Geometry: final body of the model. Coordinates: model frame, mm. A direction names the side the tool comes from. Coordinates: 2 decimals unless noted, no trailing zeros. Loops run counter-clockwise (first coordinate to the right, second up) from the corner with the lowest first, then second, coordinate; pieces in that order, holes last. Notation, with made-up numbers: M 22,89.5 L 36,89.5 A20 cw 36,125.5 Z; hole C -24,-10 d5. An arc over 180 degrees is marked long. Write item = value, one per line. Start each with the question number.
```python
from build123d import *

# Parameters (mm, degrees)
SKETCH005_AS_DRAWN_R                 = 10
EXTRUDE005_DEPTH                     = 5
EXTRUDE005_ONTO_SKETCH005_ROLL_ANGLE = 90
SKETCH001_AS_DRAWN_W                 = 40
SKETCH001_AS_DRAWN_H                 = 70
SKETCH001_AS_DRAWN_R                 = 3.5
EXTRUDE002_DEPTH                     = 12
EXTRUDE002_ONTO_SKETCH001_ROLL_ANGLE = 90
SKETCH004_AS_DRAWN_R                 = 8.5
SKETCH004_AS_DRAWN_R_2               = 3.5
EXTRUDE004_DEPTH                     = 2
EXTRUDE004_ONTO_SKETCH004_ROLL_ANGLE = 90
SKETCH003_AS_DRAWN_R                 = 5.95
SKETCH003_AS_DRAWN_R_2               = 4
EXTRUDE003_DEPTH                     = 25
EXTRUDE003_ONTO_SKETCH003_ROLL_ANGLE = 90
CYLINDER001_R                        = 16.25
CYLINDER001_DEPTH                    = 10
SKETCH_R                             = 14
EXTRUDE_DEPTH                        = 13
CYLINDER_R                           = 16.25
CYLINDER_DEPTH                       = 10
EXTRUDE001_DEPTH                     = 13


with BuildPart() as contra_nut_cut:
    # Sketch005 as drawn → Extrude005 (new)
    with BuildSketch(Plane.XY):
        Circle(SKETCH005_AS_DRAWN_R)
    extrude(amount=-EXTRUDE005_DEPTH)


with BuildPart() as contra_nut_cut_1:
    # Extrude005 onto Sketch005 roll: moved
    add(contra_nut_cut.part.rotate(Axis((0, 0, 0), (1, 0, 0)), EXTRUDE005_ONTO_SKETCH005_ROLL_ANGLE))


with BuildPart() as contra_nut_cut_2:
    # Extrude005 onto Sketch005 placement: moved
    add(contra_nut_cut_1.part)


with BuildPart() as contra_nut_cut_3:
    # Extrude005 placement: moved
    add(contra_nut_cut_2.part.moved(Location((0, 7, 0))))


with BuildPart() as nut_cut:
    # Sketch001 as drawn → Extrude002 (new)
    with BuildSketch(Plane.XY):
        Rectangle(SKETCH001_AS_DRAWN_W, SKETCH001_AS_DRAWN_H)
        Circle(SKETCH001_AS_DRAWN_R, mode=Mode.SUBTRACT)
    extrude(amount=-EXTRUDE002_DEPTH)


with BuildPart() as nut_cut_1:
    # Extrude002 onto Sketch001 roll: moved
    add(nut_cut.part.rotate(Axis((0, 0, 0), (1, 0, 0)), EXTRUDE002_ONTO_SKETCH001_ROLL_ANGLE))


with BuildPart() as nut_cut_2:
    # Extrude002 onto Sketch001 placement: moved
    add(nut_cut_1.part)

    # Cut002: cut contra-nut-cut
    add(contra_nut_cut_3.part, mode=Mode.SUBTRACT)


with BuildPart() as nut_cut_3:
    # Cut002 placement: moved
    add(nut_cut_2.part.moved(Location((0, -36, 0))))


with BuildPart() as z_bearings_pad:
    # Sketch004 as drawn → Extrude004 (new)
    with BuildSketch(Plane.XY):
        Circle(SKETCH004_AS_DRAWN_R)
        Circle(SKETCH004_AS_DRAWN_R_2, mode=Mode.SUBTRACT)
    extrude(amount=-EXTRUDE004_DEPTH)


with BuildPart() as z_bearings_pad_1:
    # Extrude004 onto Sketch004 roll: moved
    add(z_bearings_pad.part.rotate(Axis((0, 0, 0), (1, 0, 0)), EXTRUDE004_ONTO_SKETCH004_ROLL_ANGLE))


with BuildPart() as z_bearings_pad_2:
    # Extrude004 onto Sketch004 placement: moved
    add(z_bearings_pad_1.part)


with BuildPart() as z_bearings_pad_3:
    # Extrude004 placement: moved
    add(z_bearings_pad_2.part.moved(Location((0, -38, 0))))


with BuildPart() as z_bearings_cylinder:
    # Sketch003 as drawn → Extrude003 (new)
    with BuildSketch(Plane.XY):
        Circle(SKETCH003_AS_DRAWN_R)
        Circle(SKETCH003_AS_DRAWN_R_2, mode=Mode.SUBTRACT)
    extrude(amount=-EXTRUDE003_DEPTH)


with BuildPart() as z_bearings_cylinder_1:
    # Extrude003 onto Sketch003 roll: moved
    add(z_bearings_cylinder.part.rotate(Axis((0, 0, 0), (1, 0, 0)), EXTRUDE003_ONTO_SKETCH003_ROLL_ANGLE))


with BuildPart() as z_bearings_cylinder_2:
    # Extrude003 onto Sketch003 placement: moved
    add(z_bearings_cylinder_1.part)


with BuildPart() as z_bearings_cylinder_3:
    # Extrude003 placement: moved
    add(z_bearings_cylinder_2.part.moved(Location((0, -61, 0))))


with BuildPart() as cylinder001:
    # Cylinder001 → Cylinder001 (new body)
    with BuildSketch(Plane.XY.offset(3)):
        Circle(CYLINDER001_R)
    extrude(amount=CYLINDER001_DEPTH)


with BuildPart() as bearing_nest_r_cut:
    # Sketch → Extrude (new body)
    with BuildSketch(Plane.XY):
        with BuildLine():
            ThreePointArc((20, 0), (0, 20), (-20, 0))
            Line((-20, 0), (-20, -36))
            Line((-20, -36), (20, -36))
            Line((20, -36), (20, 0))
        make_face()
        Circle(SKETCH_R, mode=Mode.SUBTRACT)
    extrude(amount=EXTRUDE_DEPTH)

    # Cut001: cut Cylinder001
    add(cylinder001.part, mode=Mode.SUBTRACT)


with BuildPart() as bearing_nest_r_cut_1:
    # Cut001 placement: moved
    add(bearing_nest_r_cut.part.moved(Location((0, 0, 22))))


with BuildPart() as cylinder:
    # Cylinder → Cylinder (new body)
    with BuildSketch(Plane.XY):
        Circle(CYLINDER_R)
    extrude(amount=CYLINDER_DEPTH)


with BuildPart() as fusion:
    # Sketch → Extrude001 (new body)
    with BuildSketch(Plane.XY):
        with BuildLine():
            ThreePointArc((20, 0), (0, 20), (-20, 0))
            Line((-20, 0), (-20, -36))
            Line((-20, -36), (20, -36))
            Line((20, -36), (20, 0))
        make_face()
        Circle(SKETCH_R, mode=Mode.SUBTRACT)
    extrude(amount=EXTRUDE001_DEPTH)

    # Cut: cut Cylinder
    add(cylinder.part, mode=Mode.SUBTRACT)


with BuildPart() as fusion_1:
    # Cut placement: moved
    add(fusion.part.moved(Location((0, 0, -35))))

    # Fusion: union nut-cut, z-bearings-pad, z-bearings-cylinder, bearing-nest-r-cut
    add(nut_cut_3.part)
    add(z_bearings_pad_3.part)
    add(z_bearings_cylinder_3.part)
    add(bearing_nest_r_cut_1.part)


solid = fusion_1.part
```
Item 1: Section query B-B (x = -7). Count the separate pieces of the cut face and the enclosed holes in it, plus the area to 3 significant figures.
Item 2: Reachability of faces 5 (the flat face through (0, -16, -22)), 6 (the cylindrical face through (-0.867, -49.661, -3.905)), 7 (the flat face through (-13.3, 4.9, 25)) from +Z, -Z, +X, -X, +Y, -Y: full face, straight path, thin tool, end or side. Return the list, or none.
Item 3: Section query C-C (y = -11.5). Return the cut outline in (x, z), plus the area to 3 significant figures.
Item 4: First-contact query: pin 1 (3 mm diameter, centred on x = 12, y = -0.5, fed in from +Z) (1 decimal); pin 2 (1.5 mm diameter, centred on x = 4, z = -24, fed in from -Y); pin 3 (10 mm diameter, centred on x = 5.5, y = -49, fed in from -Z); pin 4 (3 mm diameter, centred on x = 11.5, z = -24, fed in from +Y). Flat tips, straight axial feed; report the tip coordinate or a pass-through.
Item 5: Section query A-A (z = 0). Return the cut outline in (x, y), plus the area to 3 significant figures.
Item 6: Section query D-D (z = -27). Return the cut outline in (x, y).
Item 7: Pull-direction query (Y, two-part tool) for faces 1 (the cylindrical face through (15.5, 4.88, 29.93)), 2 (the cylindrical face through (0, 20, -29)), 3 (the cylindrical face through (12.932, -5.362, 23.479)), 4 (the cylindrical face through (4.57, -37.014, 7.167)); classes: released by +Y, released by -Y, zero draft, split by the parting line, or undercut.
Item 8: Line query: line 1 (Y direction, x = 0, z = -23); line 2 (Z direction, x = -13.5, y = -19.5); line 3 (Z direction, x = 12, y = 9). Output: solid intervals per line, ascending. Write a range as from..to.
Verdict:
q1.separate_pieces = 3
q1.enclosed_holes = 0
q1.area = 1,170 mm2
q2.face_5 = +X, -X, +Y
q2.face_6 = -Y
q2.face_7 = +Z
q3.outline = M -20,-35 L -11.48,-35 L -11.48,-25 L -7.98,-25 L -7.98,-22 L -20,-22 Z; M -20,22 L -7.98,22 L -7.98,25 L -11.48,25 L -11.48,35 L -20,35 Z; M 7.98,-25 L 11.48,-25 L 11.48,-35 L 20,-35 L 20,-22 L 7.98,-22 Z; M 7.98,22 L 20,22 L 20,35 L 11.48,35 L 11.48,25 L 7.98,25 Z
q3.area = 485 mm2
q4.pin_1 = through
q4.pin_2 = -36
q4.pin_3 = -5.93
q4.pin_4 = 17.32
q5.outline = M -20,-36 L -8.5,-36 L -8.5,-38 L -5.95,-38 L -5.95,-61 L -4,-61 L -4,-38 L -3.5,-38 L -3.5,-29 L -10,-29 L -10,-24 L -20,-24 Z; M 3.5,-38 L 4,-38 L 4,-61 L 5.95,-61 L 5.95,-38 L 8.5,-38 L 8.5,-36 L 20,-36 L 20,-24 L 10,-24 L 10,-29 L 3.5,-29 Z
q5.area = 441 mm2
q6.outline = M -20,-36 L 20,-36 L 20,0 A20 ccw -20,0 Z; hole C 0,0 d32.5
q7.face_1 = undercut
q7.face_2 = released by +Y
q7.face_3 = undercut
q7.face_4 = zero draft
q8.line_1 = -36..-14, 14..20
q8.line_2 = -35..-22, 22..35
q8.line_3 = -25..-22, 22..25
